```python
from build123d import *

# Parameters (mm, degrees)
SKETCH1_W                      = 676.28516
SKETCH1_H                      = 203.2
BASE_FLANGE1_DEPTH             = 3.175
EDGE_FLANGE2_STRIP_W           = 19.05
EDGE_FLANGE2_STRIP_H           = 3.175
EDGE_FLANGE2_STRIP_CUT_DEPTH   = 203.2
EDGE_FLANGE2_STRIP_2_W         = 19.05
EDGE_FLANGE2_STRIP_2_H         = 3.175
EDGE_FLANGE2_STRIP_CUT_2_DEPTH = 203.2
EDGE_FLANGE2_DEPTH             = 203.2
EDGE_FLANGE2_BEND_DEPTH        = 203.2
EDGE_FLANGE3_DEPTH             = 434.98516


# Sheet-metal steps are written as plain solids
with BuildPart() as part:
    # Sketch1 → Base-Flange1 (new body)
    with BuildSketch(Plane(origin=(0, 0, 0), x_dir=(1, 0, 0), z_dir=(0, 1, 0))):
        with Locations((338.14258, 101.6)):
            Rectangle(SKETCH1_W, SKETCH1_H)
    extrude(amount=-BASE_FLANGE1_DEPTH)

    # Edge-Flange2 strip (across the edge) → Edge-Flange2 strip cut (cut)
    with BuildSketch(Plane(origin=(676.28516, 0, 0), x_dir=(-1, 0, 0), z_dir=(0, 0, -1))):
        with Locations((-3.175, -1.5875)):
            Rectangle(EDGE_FLANGE2_STRIP_W, EDGE_FLANGE2_STRIP_H)
    extrude(amount=EDGE_FLANGE2_STRIP_CUT_DEPTH, mode=Mode.SUBTRACT)

    # Edge-Flange2 strip 2 (across the edge) → Edge-Flange2 strip cut 2 (cut)
    with BuildSketch(Plane.XY.offset(-203.2)):
        with Locations((-3.175, -1.5875)):
            Rectangle(EDGE_FLANGE2_STRIP_2_W, EDGE_FLANGE2_STRIP_2_H)
    extrude(amount=EDGE_FLANGE2_STRIP_CUT_2_DEPTH, mode=Mode.SUBTRACT)

    # Edge-Flange2 section (across the edge) → Edge-Flange2 (add)
    with BuildSketch(Plane(origin=(676.28516, 0, 0), x_dir=(-1, 0, 0), z_dir=(0, 0, -1))):
        with BuildLine():
            Line((0, 3.175), (0, 22.225))
            Line((0, 22.225), (3.175, 22.225))
            Line((3.175, 22.225), (3.175, 3.175))
            ThreePointArc((3.175, 3.175), (4.10493597, 0.92993597), (6.35, 0))
            Line((6.35, 0), (6.35, -3.175))
            ThreePointArc((6.35, -3.175), (1.859871939, -1.315128061), (0, 3.175))
        make_face()
    extrude(amount=EDGE_FLANGE2_DEPTH)

    # Edge-Flange2 section 2 (across the edge) → Edge-Flange2 bend (add)
    with BuildSketch(Plane.XY.offset(-203.2)):
        with BuildLine():
            Line((0, 3.175), (0, 22.225))
            Line((0, 22.225), (3.175, 22.225))
            Line((3.175, 22.225), (3.175, 3.175))
            ThreePointArc((3.175, 3.175), (4.10493597, 0.92993597), (6.35, 0))
            Line((6.35, 0), (6.35, -3.175))
            ThreePointArc((6.35, -3.175), (1.859871939, -1.315128061), (0, 3.175))
        make_face()
    extrude(amount=EDGE_FLANGE2_BEND_DEPTH)

    # Edge-Flange3 section (across the edge) → Edge-Flange3 (add)
    with BuildSketch(Plane(origin=(555.63516, 0, -206.375), x_dir=(0, 0, 1), z_dir=(-1, 0, 0))):
        with BuildLine():
            Line((-3.175, 3.175), (-3.175, 34.925))
            Line((-3.175, 34.925), (0, 34.925))
            Line((0, 34.925), (0, 3.175))
            ThreePointArc((0, 3.175), (0.92993597, 0.92993597), (3.175, 0))
            Line((3.175, 0), (3.175, -3.175))
            ThreePointArc((3.175, -3.175), (-1.315128061, -1.315128061), (-3.175, 3.175))
        make_face()
    extrude(amount=EDGE_FLANGE3_DEPTH)


solid = part.part
```
Geometry check sheet. Reference: the model listing, model coordinates, mm. A direction names the side the tool comes from. Round coordinates to 2 decimals unless told otherwise and drop trailing zeros. Loops run counter-clockwise (first coordinate to the right, second up) from the corner with the lowest first, then second, coordinate; pieces in that order, holes last. Notation, with made-up numbers: M 71,3 L 119,3 A14 ccw 119,7 Z; hole C 62.5,66 d4. An arc over 180 degrees is marked long. Return JSON: item names as keys, results as strings. Group by question number.
(1) Mould release check, pull along X, two halves, no side actions. Record for faces 4 (the face through (333, -3.175, -103)), 5 (the face through (333, 0, -103)), 6 (the face through (0, 13, -103)): pulls with the +X half, pulls with the -X half, needs draft (parallel to the pull), parting line crosses it, or undercut.
(2) Scan lines: line 1 along X through (y, z) = (11, -11) (3 decimals); line 2 along Z through (x, y) = (436, 8.5) (3 decimals); line 3 along Y through (x, z) = (85, -26) (3 decimals). Record each from-to range of solid material in increasing order. Write a range as [from, to].
(3) Section check B-B, the plane z = -43.5. Enter the section's corners in (x, y) (3 decimals), and give its area (3 significant figures).
(4) Set-up check for faces 1 (the face through (673.11, 13, -100)), 2 (the face through (630, -2, -203.2)), 3 (the face through (341, 19, -206.375)): record each of +Z, -Z, +X, -X, +Y, -Y from which the full face is reachable in a straight line by a thin tool's end or side.
(5) Section check C-C, the plane x = 491. Enter the section's corners in (y, z) (3 decimals).
(6) Section check D-D, the plane x = 625.5. Enter the section's corners in (y, z) (3 decimals), and give its area (3 significant figures).
(7) Section check A-A, the plane y = 16. Enter the section's corners in (x, z) (3 decimals), and give its area (3 significant figures).
(8) Go/stop test with flat-tipped pins: pin 1 (10 mm diameter, centred on x = 294.5, z = -119, fed in from +Y); pin 2 (1.6 mm diameter, centred on x = 675, z = -81.5, fed in from +Y) (3 decimals); pin 3 (9.5 mm diameter, centred on x = 430, y = 19, fed in from +Z) (3 decimals). Record where each tip stops, or that it passes through.
Data:
{
 "1": {"face 4": "needs draft", "face 5": "undercut", "face 6": "pulls with the -X half"},
 "2": {"line 1": "[0, 3.175], [673.11, 676.285]", "line 2": "[-209.55, -206.375]", "line 3": "[-3.175, 0]"},
 "3": {"outline": "M 0,3.175 A6.35 ccw 6.35,-3.175 L 669.935,-3.175 A6.35 ccw 676.285,3.175 L 676.285,22.225 L 673.11,22.225 L 673.11,3.175 A3.175 cw 669.935,0 L 6.35,0 A3.175 cw 3.175,3.175 L 3.175,22.225 L 0,22.225 Z", "area": "2,280 mm²"},
 "4": {"face 1": "+Z, -Z, +Y", "face 2": "-Z, +X, +Y, -Y", "face 3": "+Z, +X, -X, +Y"},
 "5": {"outline": "M -3.175,-203.2 A6.35 ccw 3.175,-209.55 L 34.925,-209.55 L 34.925,-206.375 L 3.175,-206.375 A3.175 cw 0,-203.2 L 0,0 L -3.175,0 Z"},
 "6": {"outline": "M -3.175,-203.2 L 0,-203.2 L 0,0 L -3.175,0 Z", "area": "645 mm²"},
 "7": {"outline": "M 0,-203.2 L 3.175,-203.2 L 3.175,0 L 0,0 Z; M 120.65,-209.55 L 555.635,-209.55 L 555.635,-206.375 L 120.65,-206.375 Z; M 673.11,-203.2 L 676.285,-203.2 L 676.285,0 L 673.11,0 Z", "area": "2,670 mm²"},
 "8": {"pin 1": "y = 0", "pin 2": "y = 22.225", "pin 3": "z = -206.375"}
}
